```python
from build123d import *

# Parameters (mm, degrees)
SKETCH_1_W          = 109
SKETCH_1_H          = 78.25
EXTRUDE_1_DEPTH     = 5
CUT_EXTRUDE_1_DEPTH = 5
SKETCH_3_W          = 18.95
SKETCH_3_H          = 4.7
SKETCH_3_W_2        = 19.5
EXTRUDE_2_DEPTH     = 10.5
SKETCH_4_R          = 1.7
CUT_EXTRUDE_2_DEPTH = 5
SKETCH_5_R          = 1.7
CUT_EXTRUDE_3_DEPTH = 5
FILLET_1_R          = 5
FILLET_2_R          = 1
FILLET_3_R          = 1


with BuildPart() as part:
    # 草圖1 → 填料-伸長1 (new body)
    with BuildSketch(Plane.YZ):
        Rectangle(SKETCH_1_W, SKETCH_1_H)
    extrude(amount=EXTRUDE_1_DEPTH)

    # 草圖2 → 除料-伸長1 (cut)
    with BuildSketch(Plane(origin=(0, 0, 0), x_dir=(0, -1, 0), z_dir=(-1, 0, 0))):
        Polygon((-54.5, 39.125), (-54.5, -34.425), (-45, 4.475), (-45, 39.125), align=None)
        Polygon((45, 39.125), (45, 4.475), (54.5, -34.425), (54.5, 39.125), align=None)
        Polygon((-35, -34.425), (35, -34.425), (26.05, 4.475), (26.05, 19.125), (-26.05, 19.125), (-26.05, 4.475), align=None)
    extrude(amount=-CUT_EXTRUDE_1_DEPTH, mode=Mode.SUBTRACT)

    # 草圖3 → 填料-伸長2 (add)
    with BuildSketch(Plane(origin=(0, 0, 0), x_dir=(0, -1, 0), z_dir=(-1, 0, 0))):
        with Locations((-35.525, 6.825)):
            Rectangle(SKETCH_3_W, SKETCH_3_H)
        with Locations((-44.75, -36.775)):
            Rectangle(SKETCH_3_W_2, SKETCH_3_H)
        with Locations((44.75, -36.775)):
            Rectangle(SKETCH_3_W_2, SKETCH_3_H)
        with Locations((35.525, 6.825)):
            Rectangle(SKETCH_3_W, SKETCH_3_H)
    extrude(amount=EXTRUDE_2_DEPTH)

    # 草圖4 → 除料-伸長2 (cut)
    with BuildSketch(Plane(origin=(0, 0, 9.175), x_dir=(0, -1, 0), z_dir=(0, 0, 1))):
        with Locations(Location((-40, -5.5, 0), (0, 0, 90))):
            Circle(SKETCH_4_R)
        with Locations(Location((-31.05, -5.5, 0), (0, 0, 90))):
            Circle(SKETCH_4_R)
        with Locations((31.05, -5.5)):
            Circle(SKETCH_4_R)
        with Locations((40, -5.5)):
            Circle(SKETCH_4_R)
    extrude(amount=-CUT_EXTRUDE_2_DEPTH, mode=Mode.SUBTRACT)

    # 草圖5 → 除料-伸長3 (cut)
    with BuildSketch(Plane(origin=(0, 0, -34.425), x_dir=(0, -1, 0), z_dir=(0, 0, 1))):
        with Locations(Location((-49.5, -5.5, 0), (0, 0, 90))):
            Circle(SKETCH_5_R)
        with Locations(Location((-40, -5.5, 0), (0, 0, 90))):
            Circle(SKETCH_5_R)
        with Locations((40, -5.5)):
            Circle(SKETCH_5_R)
        with Locations(Location((49.5, -5.5, 0), (0, 0, 90))):
            Circle(SKETCH_5_R)
    extrude(amount=-CUT_EXTRUDE_3_DEPTH, mode=Mode.SUBTRACT)

    # 圓角1
    fillet_1_edges = [part.edges().sort_by_distance(p)[0] for p in [
        (-10.5, -45, 6.825),
        (-10.5, -26.05, 6.825),
        (-10.5, -54.5, -36.775),
        (-10.5, -35, -36.775),
        (-10.5, 54.5, -36.775),
        (-10.5, 35, -36.775),
        (-10.5, 45, 6.825),
        (-10.5, 26.05, 6.825),
    ]]
    fillet(fillet_1_edges, radius=FILLET_1_R)

    # 圓角2
    fillet_2_edges = [part.edges().sort_by_distance(p)[0] for p in [
        (2.5, 45, 39.125),
        (2.5, -45, 39.125),
    ]]
    fillet(fillet_2_edges, radius=FILLET_2_R)

    # 圓角3
    # the kernel refuses this fillet: 1 mm, written as the material it adds along each edge
    with BuildSketch(Plane(origin=(0, 35, -34.425), x_dir=(0, -1, 0), z_dir=(1, 0, 0))) as fillet_3_piece_1:
        with BuildLine():
            CenterArc((FILLET_3_R * 1.25620356602, -FILLET_3_R), FILLET_3_R, 90, 102.956961135)
            Line((FILLET_3_R * 0.281664799684, -FILLET_3_R * 1.22421907349), (0, 0))
            Line((0, 0), (FILLET_3_R * 1.25620356602, 0))
        make_face()
    extrude(amount=5)
    with BuildSketch(Plane(origin=(0, 26.05, 19.125), x_dir=(0, -1, 0), z_dir=(1, 0, 0)), Plane(origin=(0, -26.05, 19.125), x_dir=(0, 0, -1), z_dir=(1, 0, 0))) as fillet_3_piece_2:
        with BuildLine():
            CenterArc((FILLET_3_R, FILLET_3_R), FILLET_3_R, 180, 90)
            Line((0, FILLET_3_R), (0, 0))
            Line((0, 0), (FILLET_3_R, 0))
        make_face()
    extrude(amount=5)
    with BuildSketch(Plane(origin=(0, -35, -34.425), x_dir=(0, 1, 0), z_dir=(1, 0, 0))) as fillet_3_piece_3:
        with BuildLine():
            CenterArc((FILLET_3_R * 1.25620356602, FILLET_3_R), FILLET_3_R, 167.043038865, 102.956961135)
            Line((FILLET_3_R * 0.281664799684, FILLET_3_R * 1.22421907349), (0, 0))
            Line((0, 0), (FILLET_3_R * 1.25620356602, 0))
        make_face()
    extrude(amount=5)


solid = part.part
```
Input: part model. Units: mm. Frame: model coordinates. A direction names the side the tool comes from. Round coordinates to 2 decimals unless told otherwise and drop trailing zeros. Loops run counter-clockwise (first coordinate to the right, second up) from the corner with the lowest first, then second, coordinate; pieces in that order, holes last. Notation, with made-up numbers: M -29,-34 L 15,-34 A20 cw 15,-29 Z; hole C 38,-11.75 d4. An arc over 180 degrees is marked long. Answer in a Markdown table with one row per item. Add a question column.
1. Section B-B (x = -1.25). Output: boundary loops of the cut face in (y, z) (3 decimals).
2. Section D-D (z = 25). Output: boundary loops of the cut face in (x, y), and give its area (3 significant figures).
3. Section C-C (z = 16.5). Output: boundary loops of the cut face in (x, y).
4. Set-up query: faces 1 (the face through (2, 45, 21)), 2 (the face through (2, 0, 19.125)), 3 (the face through (0, 1, -36)). Return all of +Z, -Z, +X, -X, +Y, -Y with unobstructed straight access to the full face (end or side cutting, diameter ignored); none if empty.
5. Mould query, pull axis Y, two halves, no side actions, for faces 4 (the face through (-5, -35, 4.475)), 5 (the face through (-4.99, -32.67, 6.86)), 6 (the face through (2.465, 49.816, -15.247)), 7 (the face through (-4.586, 32.483, 6.858)). Classes: released by +Y, released by -Y, zero draft, split by the parting line, or undercut.
6. Ray query, probe 1 along X at (y, z) = (-31.05, 7.4); probe 2 along Z at (x, y) = (3, -11) (3 decimals); probe 3 along Y at (x, z) = (4, 6). Return the intervals inside material, ascending.
7. Contact query for flat-ended pins moving along their axis: pin 1 (8 mm diameter, centred on x = -6, z = 11, fed in from +Y); pin 2 (5.5 mm diameter, centred on x = -5.5, y = 40, fed in from +Z) (3 decimals); pin 3 (2 mm diameter, centred on x = 2, z = 3, fed in from +Y). Output: stop coordinate, or through.
8. Section A-A (y = 22.5). Output: boundary loops of the cut face in (x, z) (3 decimals), and give its area (4 significant figures).
Values follow:
| question | item | result |
|---|---|---|
| 1 | outline | M -54.5,-39.125 L -35,-39.125 L -35,-34.425 L -54.5,-34.425 Z; M -45,4.475 L -26.05,4.475 L -26.05,9.175 L -45,9.175 Z; M 26.05,4.475 L 45,4.475 L 45,9.175 L 26.05,9.175 Z; M 35,-39.125 L 54.5,-39.125 L 54.5,-34.425 L 35,-34.425 Z |
| 2 | outline | M 0,-45 L 5,-45 L 5,45 L 0,45 Z |
| 2 | area | 450 mm^2 |
| 3 | outline | M 0,-45 L 5,-45 L 5,-26.05 L 0,-26.05 Z; M 0,26.05 L 5,26.05 L 5,45 L 0,45 Z |
| 4 | face 1 | +Z, +X, -X, +Y |
| 4 | face 2 | +X, -X |
| 4 | face 3 | -X |
| 5 | face 4 | zero draft |
| 5 | face 5 | undercut |
| 5 | face 6 | released by +Y |
| 5 | face 7 | undercut |
| 6 | probe 1 | -10.5 to -7.2, -3.8 to 5 |
| 6 | probe 2 | -39.125 to -34.425, 19.125 to 39.125 |
| 6 | probe 3 | -45 to -26.05, 26.05 to 45 |
| 7 | pin 1 | y = 45 |
| 7 | pin 2 | z = 9.175 |
| 7 | pin 3 | y = 45.6 |
| 8 | outline | M 0,-39.125 L 5,-39.125 L 5,-34.425 L 0,-34.425 Z; M 0,19.125 L 5,19.125 L 5,39.125 L 0,39.125 Z |
| 8 | area | 123.5 mm^2 |
